Could you check a few things on this model? Use its own coordinates, in mm. A direction names the side the tool comes from. Round coordinates to 2 decimals unless told otherwise and drop trailing zeros. Order: outer loops, then holes, each group sorted by start corner. A loop starts at its lowest first (then second) coordinate and runs counter-clockwise, first axis right, second up. Notation, with made-up numbers: (67.25, -13) -> (79.25, -13) arc R28 ccw to (79.25, 26) -> close; hole circle Ø3 at (44.25, 82.5). An arc over 180 degrees is marked (long way). One line per question, with ' | ' between items.
```python
from build123d import *

# Parameters (mm, degrees)
F1_ANGLE = 90
F2_DEPTH = 2
F3_DEPTH = 0.25
F4_DEPTH = 0.25


with BuildPart() as f1:
    # F0 (on Right) → F1 (revolve)
    with BuildSketch(Plane.YZ):
        Polygon((4.25, 5), (3.75, 2.5), (5.25, 2.5), (5.25, 5), align=None)
    revolve(axis=Axis((0, 0, 2.5), (0, 0, 1)), revolution_arc=F1_ANGLE)

    # F2 (add): a face of the model
    f2_faces = [f1.faces().sort_by_distance(p)[0] for p in [
        (-2.8913147995, 2.8913147995, 2.5),
    ]]
    extrude(f2_faces, amount=F2_DEPTH)

    # F3 (add): a face of the model
    f3_faces = [f1.faces().sort_by_distance(p)[0] for p in [
        (0, 4.5595238095, 2.6054421769),
    ]]
    extrude(f3_faces, amount=F3_DEPTH)

    # F4 (add): a face of the model
    f4_faces = [f1.faces().sort_by_distance(p)[0] for p in [
        (-4.5595238095, 0, 2.6054421769),
    ]]
    extrude(f4_faces, amount=F4_DEPTH)

    # F5: F1 across face


with BuildPart() as f1_1:
    add(f1.part)
    add(f1.part.mirror(Plane(origin=(-4.5595238095, -0.25, 2.6054421769), x_dir=(1, 0, 0), z_dir=(0, -1, 0))))

    # F6: F1 across face


with BuildPart() as f1_2:
    add(f1_1.part)
    add(f1_1.part.mirror(Plane(origin=(0.25, -5.0595238095, 2.6054421769), x_dir=(0, 1, 0), z_dir=(1, 0, 0))))


solid = f1_2.part
```
1. I need wall thicknesses on probe 1 along X at (y, z) = (-1.5, 2.1); probe 2 along Y at (x, z) = (-0.5, 1.85); probe 3 along Y at (x, z) = (-1, 4.5). Which ranges of each line are inside material? Lowest first, please.
From the geometry:
probe 1: x = -5.15 to -3.61, 4.11 to 5.65 | probe 2: y = -5.73 to -4.22, 3.72 to 5.23 | probe 3: y = -5.65 to -4.53, 4.03 to 5.15
2. I want a section at A-A on z = 4.2. List the corners of the cut face in (x, y) for me, and give its area (3 significant figures).
From the geometry:
outline: (-5.25, -0.5) arc R5.25 ccw to (0, -5.75) -> (0.5, -5.75) arc R5.25 ccw to (5.75, -0.5) -> (5.75, 0) arc R5.25 ccw to (0.5, 5.25) -> (0, 5.25) arc R5.25 ccw to (-5.25, 0) -> close; hole (-4.09, -0.5) arc R4.09 ccw to (0, -4.59) -> (0.5, -4.59) arc R4.09 ccw to (4.59, -0.5) -> (4.59, 0) arc R4.09 ccw to (0.5, 4.09) -> (0, 4.09) arc R4.09 ccw to (-4.09, 0) -> close | area: 36.4 mm²
3. If we mould it in two halves opening along X, with no side actions, what happens to faces 4 (the face through (-3, -3, 0.5)), 5 (the face through (3.29, 2.86, 3.73)), 6 (the face through (-3.671, -4.253, 2.782)), 7 (the face through (3.1, -3.2, 1.5))? For each: pulls with the +X half, pulls with the -X half, needs draft (parallel to the pull), parting line crosses it, or undercut.
From the geometry:
face 4: needs draft | face 5: undercut | face 6: pulls with the -X half | face 7: undercut
4. I'm going to push flat-ended pins straight in: pin 1 (2 mm diameter, centred on x = -3, z = 2, fed in from +Y); pin 2 (1.5 mm diameter, centred on x = -3.5, z = 2.5, fed in from +Y). Where does each tip first touch, or does it pass through?
From the geometry:
pin 1: stops at y = 4.85 | pin 2: stops at y = 4.47
5. On a 3-axis mill with a long thin cutter (end or side, diameter ignored), from which of +Z, -Z, +X, -X, +Y, -Y can I reach the whole of each face in a straight line? I mean faces 1 (the face through (4.171, 3.753, 2.782)), 2 (the face through (3.29, -3.36, 3.73)), 3 (the face through (-2.6, 2.7, 1.5)). Say none if no direction works.
From the geometry:
face 1: +Z, -Z, +X, +Y | face 2: +Z | face 3: +Z, -Z
6. I want a section at B-B on z = 2.2. List the corners of the cut face in (x, y) for me, and give its area (3 significant figures).
From the geometry:
outline: (-5.25, -0.5) arc R5.25 ccw to (0, -5.75) -> (0.5, -5.75) arc R5.25 ccw to (5.75, -0.5) -> (5.75, 0) arc R5.25 ccw to (0.5, 5.25) -> (0, 5.25) arc R5.25 ccw to (-5.25, 0) -> close; hole (-3.75, -0.5) arc R3.75 ccw to (0, -4.25) -> (0.5, -4.25) arc R3.75 ccw to (4.25, -0.5) -> (4.25, 0) arc R3.75 ccw to (0.5, 3.75) -> (0, 3.75) arc R3.75 ccw to (-3.75, 0) -> close | area: 45.4 mm²
